```python
from build123d import *

# Parameters (mm, degrees)
EXTRUDE_1_DEPTH     = 17
EXTRUDE_2_DEPTH     = 2.1
EXTRUDE_3_DEPTH     = 2.1
CUT_EXTRUDE_1_DEPTH = 32.771213386
CUT_EXTRUDE_2_DEPTH = 32.771213386


with BuildPart() as part:
    # 草图1 → 凸台-拉伸1 (new body)
    with BuildSketch(Plane.XY):
        Polygon((0, 0), (20, 0), (20, 2.1), (2.1, 2.1), (2.1, 20), (0, 20), align=None)
    extrude(amount=EXTRUDE_1_DEPTH)

    # 草图2 → 凸台-拉伸2 (add)
    with BuildSketch(Plane(origin=(0, 0, 0), x_dir=(-1, 0, 0), z_dir=(0, 0, -1))):
        Polygon((-2.1, 20), (-2.1, 2.1), (-20, 2.1), align=None)
    extrude(amount=-EXTRUDE_2_DEPTH)

    # 草图3 → 凸台-拉伸3 (add)
    with BuildSketch(Plane.XY.offset(17)):
        Polygon((2.1, 20), (2.1, 2.1), (20, 2.1), align=None)
    extrude(amount=-EXTRUDE_3_DEPTH)

    # 草图4 → 切除-拉伸1 (cut, through all)
    with BuildSketch(Plane(origin=(2.1, 0, 0), x_dir=(0, 0, -1), z_dir=(1, 0, 0))):
        with BuildLine():
            Line((-11.5, 13.5), (-11.5, 8.5))
            ThreePointArc((-11.5, 8.5), (-8.5, 5.5), (-5.5, 8.5))
            Line((-5.5, 8.5), (-5.5, 13.5))
            ThreePointArc((-5.5, 13.5), (-8.5, 16.5), (-11.5, 13.5))
        make_face()
    extrude(amount=-CUT_EXTRUDE_1_DEPTH, mode=Mode.SUBTRACT)

    # 草图5 → 切除-拉伸2 (cut, through all)
    with BuildSketch(Plane(origin=(0, 2.1, 0), x_dir=(1, 0, 0), z_dir=(0, 1, 0))):
        with BuildLine():
            Line((8.5, -11.5), (13.5, -11.5))
            ThreePointArc((13.5, -11.5), (16.5, -8.5), (13.5, -5.5))
            Line((13.5, -5.5), (8.5, -5.5))
            ThreePointArc((8.5, -5.5), (5.5, -8.5), (8.5, -11.5))
        make_face()
    extrude(amount=-CUT_EXTRUDE_2_DEPTH, mode=Mode.SUBTRACT)


solid = part.part
```
Here's how the part is built. I have some questions about the finished solid (model axes, mm). A direction names the side the tool comes from. Give positions to 0.01 mm unless a question says otherwise; leave off trailing zeros. Loops run counter-clockwise (first coordinate to the right, second up) from the corner with the lowest first, then second, coordinate; pieces in that order, holes last. Notation, with made-up numbers: (21.5, -7.75) -> (28.5, -7.75) arc R15 ccw to (28.5, 16.25) -> close; hole circle Ø7 at (55, 85.5). An arc over 180 degrees is marked (long way). Use one line per item in the form item = value. Start each with the question number.
1) Imagine slicing it at D-D (x = 3.25). Please give me the cut outline in (y, z), then the cut area to 3 significant figures.
2) For P1, Ø4, axis at x = 3.5, y = 14.5, coming from the -Z side; P2, Ø1, axis at y = 11, z = 4.5, coming from the +X side; P3, Ø3, axis at x = 12, z = 10.5, coming from the +Y side, each with a flat end and sliding along its axis, tell me the tip position at first contact or that it passes through.
3) Imagine slicing it at B-B (y = 11). Please give me the cut outline in (x, z).
4) Please list where these lines run through material, in increasing order: line 1 along Z through (x, y) = (6.25, 7.5); line 2 along X through (y, z) = (2.25, 8.5).
5) Thinking about a two-plate mould opening in Y: for faces 1 (the face through (11.2, 10.9, 1)), 2 (the face through (1.1, 16.5, 8.4)), 3 (the face through (11, 1, 5.5)), 4 (the face through (1, 11, 5.5)), which applies, +Y half, -Y half, draft (parallel to the pull), parting line (faces both ways), or undercut?
6) Imagine slicing it at C-C (z = 8.5). Please give me the cut outline in (x, y).
7) Which directions (+Z, -Z, +X, -X, +Y, -Y) give clear straight access to the entire face, cutting with the end or side of a thin tool? Please do faces 5 (the face through (1, 11, 11.5)), 6 (the face through (16.5, 1.1, 8.6)), 7 (the face through (7, 7, 14.9)).
8) Imagine slicing it at A-A (x = 12). Please give me the cut outline in (y, z).
Check values:
q1.outline = (0, 0) -> (18.85, 0) -> (18.85, 2.1) -> (2.1, 2.1) -> (2.1, 14.9) -> (18.85, 14.9) -> (18.85, 17) -> (0, 17) -> close
q1.area = 106 mm^2
q2.P1 = 0
q2.P2 = 2.1
q2.P3 = 2.1
q3.outline = (0, 0) -> (11.1, 0) -> (11.1, 2.1) -> (2.1, 2.1) -> (2.1, 5.5) -> (0, 5.5) -> close; (0, 11.5) -> (2.1, 11.5) -> (2.1, 14.9) -> (11.1, 14.9) -> (11.1, 17) -> (0, 17) -> close
q4.line_1 = 0 to 2.1, 14.9 to 17
q4.line_2 = 0 to 2.1
q5.face_1 = +Y half
q5.face_2 = undercut
q5.face_3 = draft
q5.face_4 = undercut
q6.outline = (0, 0) -> (5.5, 0) -> (5.5, 2.1) -> (2.1, 2.1) -> (2.1, 5.5) -> (0, 5.5) -> close; (0, 16.5) -> (2.1, 16.5) -> (2.1, 20) -> (0, 20) -> close; (16.5, 0) -> (20, 0) -> (20, 2.1) -> (16.5, 2.1) -> close
q7.face_5 = +X, -X
q7.face_6 = +Y, -Y
q7.face_7 = +X, +Y
q8.outline = (0, 0) -> (10.1, 0) -> (10.1, 2.1) -> (2.1, 2.1) -> (2.1, 5.5) -> (0, 5.5) -> close; (0, 11.5) -> (2.1, 11.5) -> (2.1, 14.9) -> (10.1, 14.9) -> (10.1, 17) -> (0, 17) -> close
